Verification items for the finished model (mm, model axes). A direction names the side the tool comes from. Give positions to 0.01 mm unless a question says otherwise; leave off trailing zeros. Order: outer loops, then holes, each group sorted by start corner. A loop starts at its lowest first (then second) coordinate and runs counter-clockwise, first axis right, second up. Notation, with made-up numbers: (62, 89.25) -> (109, 89.25) arc R17 cw to (109, 121.25) -> close; hole circle Ø2 at (75.25, -37). An arc over 180 degrees is marked (long way). Return JSON: item names as keys, results as strings. Group by question number.
(1) Release check for a two-part mould opening along Y. For faces 6 (the face through (0, 0, 4.7)), 7 (the face through (-7.1, -2.89, 3.99)), 8 (the face through (12.5, 0, 1)) record: pulls with the +Y half, pulls with the -Y half, needs draft (parallel to the pull), parting line crosses it, or undercut.
(2) Tool access check on faces 1 (the face through (3, 0.5, -2)), 2 (the face through (-8, 0, 4)), 3 (the face through (0, 3.75, 4)), 4 (the face through (0, 4, -2)), 5 (the face through (7.14, -2.85, 3.99)). Record the directions out of +Z, -Z, +X, -X, +Y, -Y that give a thin tool (end or side, any length) a straight path to the whole face; none if there is none.
(3) Thickness scan on line 1 along Y through (x, z) = (0, -0.5); line 2 along Y through (x, z) = (0, 2.5); line 3 along Z through (x, y) = (6, -2). Record the ranges inside material, lowest first.
(4) Cross-section at A-A on z = -3. Enter the section's corners in (x, y), then the cut area to 3 significant figures.
(5) Cross-section at B-B on x = 0. Enter the section's corners in (y, z), then the cut area to 3 significant figures.
(6) Cross-section at C-C on y = 0. Enter the section's corners in (x, z), then the cut area to 3 significant figures.
(7) Cross-section at D-D on z = 4.25. Enter the section's corners in (x, y).
(8) Depth check by flat-ended pin: pin 1 Ø1.6 at (x, z) = (0.5, 4) entering from -Y; pin 2 Ø1.2 at (y, z) = (0, 4.5) entering from +X; pin 3 Ø1 at (x, z) = (1.5, 4) entering from +Y; pin 4 Ø2 at (x, z) = (-5.5, -3) entering from +Y. Enter the tip coordinate at first touch or a pass-through.
from build123d import *

# Parameters (mm, degrees)
SKICA1_W                 = 25
SKICA1_H                 = 10
P_IDAT_VYSUNUT_M1_DEPTH  = 3
P_IDAT_VYSUNUT_M2_DEPTH  = 2
P_IDAT_VYSUNUT_M3_DEPTH  = 4
SKICA4_R                 = 2.6
ODEBRAT_VYSUNUT_M1_DEPTH = 8.7


with BuildPart() as part:
    # Skica1 → Přidat vysunutím1 (new body)
    with BuildSketch(Plane.XY):
        Rectangle(SKICA1_W, SKICA1_H)
    extrude(amount=P_IDAT_VYSUNUT_M1_DEPTH)

    # Skica2 → Přidat vysunutím2 (add)
    with BuildSketch(Plane.XY.offset(3)):
        with BuildLine():
            Line((-5, 3.75), (5, 3.75))
            ThreePointArc((5, 3.75), (7.121320344, 2.871320344), (8, 0.75))
            Line((8, 0.75), (8, -0.75))
            ThreePointArc((8, -0.75), (7.121320344, -2.871320344), (5, -3.75))
            Line((5, -3.75), (-5, -3.75))
            ThreePointArc((-5, -3.75), (-7.121320344, -2.871320344), (-8, -0.75))
            Line((-8, -0.75), (-8, 0.75))
            ThreePointArc((-8, 0.75), (-7.121320344, 2.871320344), (-5, 3.75))
        make_face()
    extrude(amount=P_IDAT_VYSUNUT_M2_DEPTH)

    # Skica3 → Přidat vysunutím3 (add)
    with BuildSketch(Plane(origin=(0, 0, 0), x_dir=(-1, 0, 0), z_dir=(0, 0, -1))):
        with BuildLine():
            ThreePointArc((3.968626967, 0.5), (0, 4), (-3.968626967, 0.5))
            Line((-3.968626967, 0.5), (3.968626967, 0.5))
        make_face()
        with BuildLine():
            ThreePointArc((-3.968626967, -0.5), (0, -4), (3.968626967, -0.5))
            Line((3.968626967, -0.5), (-3.968626967, -0.5))
        make_face()
    extrude(amount=P_IDAT_VYSUNUT_M3_DEPTH)

    # Skica4 → Odebrat vysunutím1 (cut)
    with BuildSketch(Plane(origin=(0, 0, -4), x_dir=(-1, 0, 0), z_dir=(0, 0, -1))):
        Circle(SKICA4_R)
    extrude(amount=-ODEBRAT_VYSUNUT_M1_DEPTH, mode=Mode.SUBTRACT)


solid = part.part
Verdict:
{
 "1": {"face 6": "undercut", "face 7": "pulls with the -Y half", "face 8": "needs draft"},
 "2": {"face 1": "-Z, +X, -X", "face 2": "+Z, -X, +Y, -Y", "face 3": "+Z, +X, -X, +Y", "face 4": "-Z, +Y", "face 5": "+Z, +X, -Y"},
 "3": {"line 1": "-4 to -2.6, 2.6 to 4", "line 2": "-5 to -2.6, 2.6 to 5", "line 3": "0 to 5"},
 "4": {"outline": "(-3.97, -0.5) arc R4 ccw to (3.97, -0.5) -> (2.55, -0.5) arc R2.6 cw to (-2.55, -0.5) -> close; (-3.97, 0.5) -> (-2.55, 0.5) arc R2.6 cw to (2.55, 0.5) -> (3.97, 0.5) arc R4 ccw to start", "area": "26.2 mm²"},
 "5": {"outline": "(-5, 0) -> (-4, 0) -> (-4, -4) -> (-2.6, -4) -> (-2.6, 4.7) -> (2.6, 4.7) -> (2.6, -4) -> (4, -4) -> (4, 0) -> (5, 0) -> (5, 3) -> (3.75, 3) -> (3.75, 5) -> (-3.75, 5) -> (-3.75, 3) -> (-5, 3) -> close", "area": "31.8 mm²"},
 "6": {"outline": "(-12.5, 0) -> (-2.6, 0) -> (-2.6, 4.7) -> (2.6, 4.7) -> (2.6, 0) -> (12.5, 0) -> (12.5, 3) -> (8, 3) -> (8, 5) -> (-8, 5) -> (-8, 3) -> (-12.5, 3) -> close", "area": "82.6 mm²"},
 "7": {"outline": "(-8, -0.75) arc R3 ccw to (-5, -3.75) -> (5, -3.75) arc R3 ccw to (8, -0.75) -> (8, 0.75) arc R3 ccw to (5, 3.75) -> (-5, 3.75) arc R3 ccw to (-8, 0.75) -> close; hole circle Ø5.2 at (0, 0)"},
 "8": {"pin 1": "y = -3.75", "pin 2": "x = 8", "pin 3": "y = 3.75", "pin 4": "through"}
}
